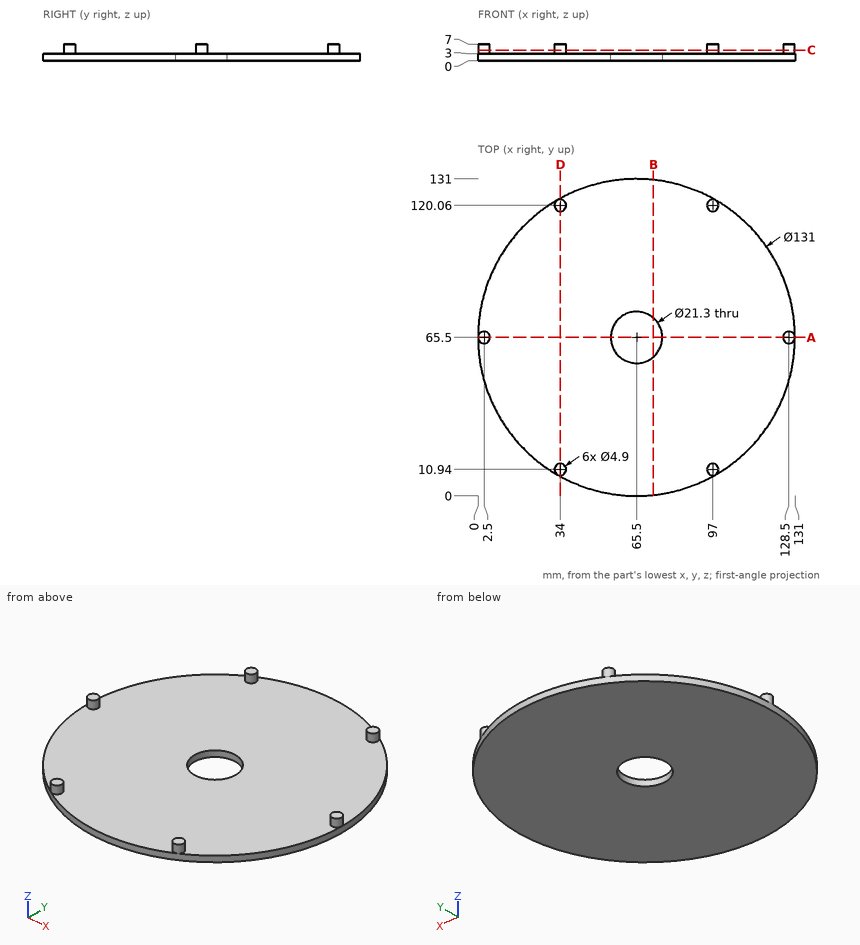
Verification items for this drawing (mm, ordinates from the low corner). Give positions to 0.01 mm unless a question says otherwise; leave off trailing zeros. Write each loop counter-clockwise with the first axis right and the second up, starting at its lowest first coordinate (ties: lowest second). Pieces come first, ordered by that corner, then holes.
1) Section check D-D, the plane x = 34. Record the boundary of the cut face in (y, z), and give its area (3 significant figures).
2) Section check A-A, the plane y = 65.5. Record the boundary of the cut face in (x, z).
3) Gauge pin test, flat end, axial feed: pin 1 (2 mm diameter, centred on x = 49, y = 97, fed in from +Z). Record the tip position at first contact, or that the pin passes through.
4) Section check B-B, the plane x = 72.5. Record the boundary of the cut face in (y, z) (1 decimal).
5) Material ranges on L1, parallel to Y at x = 65.5, z = 2.2; L2, parallel to Z at x = 87, y = 21; L3, parallel to Y at x = 77.5, z = 2, recorded low to high.
6) Section check C-C, the plane z = 4.5. Record the boundary of the cut face in (x, y), and give its area (3 significant figures).
Computed:
1. outline: (8.07, 0) - (122.93, 0) - (122.93, 3) - (122.51, 3) - (122.51, 7) - (117.61, 7) - (117.61, 3) - (13.39, 3) - (13.39, 7) - (8.49, 7) - (8.49, 3) - (8.07, 3) - close
1. area: 384 mm2
2. outline: (0, 0) - (54.85, 0) - (54.85, 3) - (4.95, 3) - (4.95, 7) - (0.05, 7) - (0.05, 3) - (0, 3) - close; (76.15, 0) - (131, 0) - (131, 3) - (130.95, 3) - (130.95, 7) - (126.05, 7) - (126.05, 3) - (76.15, 3) - close
3. pin 1: stops at z = 3
4. outline: (0.4, 0) - (57.5, 0) - (57.5, 3) - (0.4, 3) - close; (73.5, 0) - (130.6, 0) - (130.6, 3) - (73.5, 3) - close
5. L1: y = 0 to 54.85, 76.15 to 131
5. L2: z = 0 to 3
5. L3: y = 1.11 to 129.89
6. outline: circle Ø4.9 at (2.5, 65.5); circle Ø4.9 at (34, 10.94); circle Ø4.9 at (34, 120.06); circle Ø4.9 at (97, 10.94); circle Ø4.9 at (97, 120.06); circle Ø4.9 at (128.5, 65.5)
6. area: 113 mm2
